Geometry check sheet. Reference: the model listing, model coordinates, mm. A direction names the side the tool comes from. Give positions to 0.01 mm unless a question says otherwise; leave off trailing zeros. Loops run counter-clockwise (first coordinate to the right, second up) from the corner with the lowest first, then second, coordinate; pieces in that order, holes last. Notation, with made-up numbers: (73, 22.5) -> (130, 22.5) arc R29 cw to (130, 52.5) -> close; hole circle Ø3 at (-2.5, 55.5). An arc over 180 degrees is marked (long way). Answer as a JSON object with one key per item and string values.
from build123d import *

# Parameters (mm, degrees)
F0_W     = 60
F0_H     = 45
F1_DEPTH = 25
F2_R     = 18.230112
F3_DEPTH = 45.001
F4_R     = 5
F5_T     = -1


with BuildPart() as f1:
    # F0 (on Top) → F1 (new body)
    with BuildSketch(Plane.XY):
        with Locations((31.256983, 22.5)):
            Rectangle(F0_W, F0_H)
    extrude(amount=F1_DEPTH)

    # F2 (on face) → F3 (cut, through all)
    with BuildSketch(Plane.XZ):
        with Locations((61.256983, 25)):
            Circle(F2_R)
    extrude(amount=-F3_DEPTH, mode=Mode.SUBTRACT)

    # F4
    f4_edges = [f1.edges().sort_by_distance(p)[0] for p in [
        (43.026871, 22.5, 25),
        (22.141927, 0, 25),
        (1.256983, 22.5, 25),
        (22.141927, 45, 25),
    ]]
    fillet(f4_edges, radius=F4_R)

    # F5
    f5_openings = [f1.faces().sort_by_distance(p)[0] for p in [
        (31.256983, 22.5, 0),
    ]]
    offset(amount=F5_T, openings=f5_openings)


solid = f1.part
1) Section check B-B on y = 24.5. Record the cut outline in (x, z), plus the area to 3 significant figures.
Geometry check:
{"outline": "(1.26, 0) -> (2.26, 0) -> (2.26, 20) arc R4 cw to (6.26, 24) -> (38.57, 24) arc R4 cw to (42.48, 20.86) arc R19.23 ccw to (60.26, 5.8) -> (60.26, 0) -> (61.26, 0) -> (61.26, 6.77) arc R18.23 cw to (43.45, 21.08) arc R5 ccw to (38.57, 25) -> (6.26, 25) arc R5 ccw to (1.26, 20) -> close", "area": "96.6 mm2"}
2) Draft check along Y on faces 1 (the face through (22.756, 42.859, 22.797)), 2 (the face through (49.7, 22.2, 10.9)), 3 (the face through (23, 1, 23)). Enter one of: pulls with the +Y half, pulls with the -Y half, needs draft (parallel to the pull), parting line crosses it, or undercut.
Geometry check:
{"face 1": "undercut", "face 2": "needs draft", "face 3": "pulls with the -Y half"}
3) Section check D-D on z = 13.75. Record the cut outline in (x, y).
Geometry check:
{"outline": "(1.26, 0) -> (46.91, 0) -> (46.91, 45) -> (1.26, 45) -> close; hole (2.26, 1) -> (45.66, 1) -> (45.66, 44) -> (2.26, 44) -> close"}
4) Material ranges on line 1 along Y through (x, z) = (18, 19.25); line 2 along X through (y, z) = (32, 3.5); line 3 along Z through (x, y) = (16.5, 40), recorded low to high. Write a range as from..to.
Geometry check:
{"line 1": "y = 0..1, 44..45", "line 2": "x = 1.26..2.26, 60.26..61.26", "line 3": "z = 24..25"}
5) Tool access check on faces 4 (the face through (22.756, 2.141, 22.797)), 5 (the face through (2, 23, 0)). Record the directions out of +Z, -Z, +X, -X, +Y, -Y that give a thin tool (end or side, any length) a straight path to the whole face; none if there is none.
Geometry check:
{"face 4": "-Z", "face 5": "-Z, +X, -X, +Y, -Y"}
6) Depth check by flat-ended pin: P1, Ø6, axis at x = 46, y = 32, coming from the -Z side; P2, Ø3, axis at y = 6, z = 22, coming from the -X side; P3, Ø1, axis at x = 53, z = 9.5, coming from the +Y side (3 decimals); P4, Ø10, axis at x = 54.5, y = 40, coming from the +Z side. Enter the tip coordinate at first touch or a pass-through.
Geometry check:
{"P1": "stops at z = 10.18", "P2": "stops at x = 1.28", "P3": "passes through", "P4": "stops at z = 11.07"}
7) Section check C-C on x = 37. Record the cut outline in (y, z).
Geometry check:
{"outline": "(0, 0) -> (1, 0) -> (1, 20) arc R4 cw to (5, 24) -> (40, 24) arc R4 cw to (44, 20) -> (44, 0) -> (45, 0) -> (45, 20) arc R5 ccw to (40, 25) -> (5, 25) arc R5 ccw to (0, 20) -> close"}
8) Section check A-A on z = 3.25. Record the cut outline in (x, y).
Geometry check:
{"outline": "(1.26, 0) -> (61.26, 0) -> (61.26, 45) -> (1.26, 45) -> close; hole (2.26, 1) -> (60.26, 1) -> (60.26, 44) -> (2.26, 44) -> close"}
